For this review, take the finished solid that the model builds, in its own axes (mm). A direction names the side the tool comes from. Coordinates: 2 decimals unless noted, no trailing zeros. Write each loop counter-clockwise with the first axis right and the second up, starting at its lowest first coordinate (ties: lowest second). Pieces come first, ordered by that corner, then holes. Notation, with made-up numbers: (8.25, 73.25) - (39.25, 73.25) arc R10 ccw to (39.25, 85.25) - close; hole circle Ø7 at (51, 41.25). An arc over 180 degrees is marked (long way). Use one line per item in the form item = value. Start each with the question number.
1) Insertion check: P1, Ø19, axis at x = 18, y = 6, coming from the +Z side; P2, Ø4, axis at y = -7, z = 55, coming from the +X side; P3, Ø1, axis at y = -10.5, z = 24.5, coming from the +X side. Each pin has a flat end and moves straight along its axis. Give the tip position at first contact, or say it passes through.
2) We need section B-B (y = -20.5). Give the boundary of the cut face in (x, z), plus the area to 3 significant figures.
3) We need section C-C (x = 72). Give the boundary of the cut face in (y, z).
4) Tool access review of faces 1 (the flat face through (76.2, -16, 26)), 2 (the flat face through (19, 0, 63.5)), 3 (the flat face through (69, 5, 0)), 4 (the flat face through (101.6, 3, 51)), 5 (the flat face through (87, 12.7, 55)): name each direction out of +Z, -Z, +X, -X, +Y, -Y from which nothing blocks a thin tool from reaching the whole face with its end or side.
5) For L1, parallel to Y at x = 92, z = 41; L2, parallel to X at y = 5.5, z = 42; L3, parallel to X at y = 4.5, z = 47, list the stretches that pass through material, from the lowest coordinate up. Write a range as from..to.
6) We need section D-D (z = 10). Give the boundary of the cut face in (x, y) (3 decimals).
7) We need section A-A (z = 58.5). Give the boundary of the cut face in (x, y) (3 decimals).
8) Mouldability with a two-part tool opening along X and no side actions: class faces 6 (the flat face through (63.5, 3, 63)), 7 (the cylindrical face through (95.103, 4.129, 35.414)), 8 (the flat face through (108.04, 9.3, 28.53)), 9 (the flat face through (83, 3, 69.85)) as pulls with the +X half, pulls with the -X half, needs draft (parallel to the pull), parting line crosses it, or undercut.
```python
from build123d import *

# Parameters (mm, degrees)
F1_DEPTH = 25.4
F3_DEPTH = 19.05
F5_DEPTH = 12.7
F6_R     = 3.175
F7_DEPTH = 69.851


with BuildPart() as f1:
    # F0 (on Front) → F1 (new body, symmetric)
    with BuildSketch(Plane.XZ):
        Polygon((0, 63.5), (0, 25.4), (25.4, 0), (76.2, 0), (76.2, 50.8), (63.5, 55.033333), (38.1, 63.5), align=None)
        Polygon((76.2, 50.8), (76.2, 0), (114.3, 0), (114.3, 25.4), (101.6, 31.75), (101.6, 69.85), (76.2, 69.85), align=None)
        Polygon((63.5, 55.033333), (76.2, 50.8), (76.2, 69.85), (63.5, 69.85), align=None)
    extrude(amount=F1_DEPTH, both=True)

    # F2 (on face) → F3 (cut)
    with BuildSketch(Plane.XZ.offset(25.4)):
        Polygon((76.2, 0), (114.3, 0), (114.3, 25.4), (101.6, 31.75), (101.6, 69.85), (63.5, 69.85), (63.5, 55.033333), (76.2, 50.8), align=None)
    extrude(amount=-F3_DEPTH, mode=Mode.SUBTRACT)

    # F4 (on face) → F5 (cut)
    with BuildSketch(Plane(origin=(0, 25.4, 0), x_dir=(-1, 0, 0), z_dir=(0, 1, 0))):
        Polygon((-101.6, 69.85), (-101.6, 31.75), (-63.5, 55.033333), (-63.5, 69.85), align=None)
    extrude(amount=-F5_DEPTH, mode=Mode.SUBTRACT)

    # F6 (on face) → F7 (cut, through all)
    with BuildSketch(Plane.XY.offset(69.85)):
        with Locations((73.025, 3.175)):
            Circle(F6_R)
        with Locations((92.075, 3.175)):
            Circle(F6_R)
    extrude(amount=-F7_DEPTH, mode=Mode.SUBTRACT)


solid = f1.part
```
Determined:
q1.P1 = 63.5
q1.P2 = 101.6
q1.P3 = 76.2
q2.outline = (0, 25.4) - (25.4, 0) - (76.2, 0) - (76.2, 50.8) - (38.1, 63.5) - (0, 63.5) - close
q2.area = 4,270 mm²
q3.outline = (-25.4, 0) - (0.17, 0) - (0.17, 69.85) - (-6.35, 69.85) - (-6.35, 52.2) - (-25.4, 52.2) - close; (6.18, 0) - (25.4, 0) - (25.4, 49.84) - (12.7, 49.84) - (12.7, 69.85) - (6.18, 69.85) - close
q4.face_1 = +Z, -Z, +X, -Y
q4.face_2 = +Z, -X, +Y, -Y
q4.face_3 = -Z, +X, -X, +Y, -Y
q4.face_4 = +Z, +X, +Y, -Y
q4.face_5 = +Z, +X, +Y
q5.L1 = -6.35..0, 6.35..12.7
q5.L2 = 0..70.86, 75.19..89.91, 94.24..101.6
q5.L3 = 0..70.14, 75.91..89.19, 94.96..101.6
q6.outline = (15.4, -25.4) - (76.2, -25.4) - (76.2, -6.35) - (114.3, -6.35) - (114.3, 25.4) - (15.4, 25.4) - close; hole circle Ø6.35 at (73.025, 3.175); hole circle Ø6.35 at (92.075, 3.175)
q7.outline = (0, -25.4) - (53.1, -25.4) - (53.1, 25.4) - (0, 25.4) - close; (63.5, -6.35) - (101.6, -6.35) - (101.6, 12.7) - (63.5, 12.7) - close; hole circle Ø6.35 at (73.025, 3.175); hole circle Ø6.35 at (92.075, 3.175)
q8.face_6 = undercut
q8.face_7 = undercut
q8.face_8 = pulls with the +X half
q8.face_9 = needs draft
